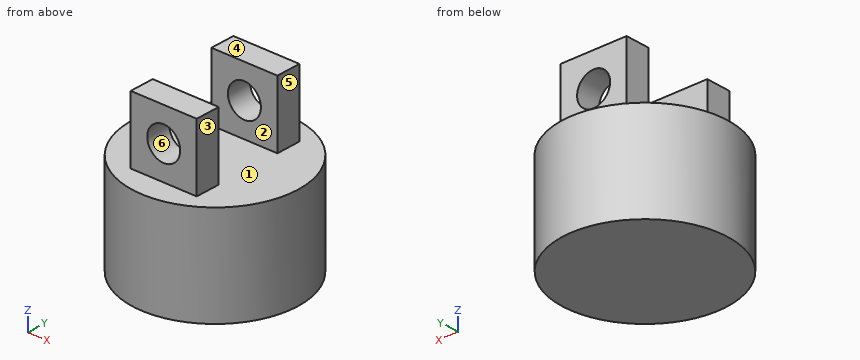
```python
from build123d import *

# Parameters (mm, degrees)
F0_R     = 31.75
F1_DEPTH = 38.1
F2_W     = 25.4
F2_H     = 9.525
F3_DEPTH = 25.4
F4_R     = 6.35
F5_DEPTH = 44.45


with BuildPart() as f1:
    # F0 (on Top) → F1 (new body)
    with BuildSketch(Plane.XY):
        Circle(F0_R)
    extrude(amount=F1_DEPTH)

    # F2 (on face) → F3 (join)
    with BuildSketch(Plane.XY.offset(38.1)):
        with Locations((0, 17.4625)):
            Rectangle(F2_W, F2_H)
        with Locations((0, -17.4625)):
            Rectangle(F2_W, F2_H)
    extrude(amount=F3_DEPTH)

    # F4 (on face) → F5 (cut, through all)
    with BuildSketch(Plane.XZ.offset(22.225)):
        with Locations((0, 50.8)):
            Circle(F4_R)
    extrude(amount=-F5_DEPTH, mode=Mode.SUBTRACT)


solid = f1.part
```
Check sheet for the modelled part. Datum: model origin and axes. Units: mm. Face numbers are marked on the shaded views. A direction names the side the tool comes from. Give positions to 0.01 mm unless a question says otherwise; leave off trailing zeros. Order: outer loops, then holes, each group sorted by start corner. A loop starts at its lowest first (then second) coordinate and runs counter-clockwise, first axis right, second up. Notation, with made-up numbers: M -27.75,-4 L 15.25,-4 A34 ccw 15.25,32 Z; hole C 9.25,15 d2. An arc over 180 degrees is marked long. Answer in a Markdown table with one row per item. Add a question column.
Q1. Access from +Z, -Z, +X, -X, +Y, -Y to the whole of each face (thin tool, end or side, straight path). Record for the marked faces 1, 2 and 3.
Q2. Gauge pin test, flat ends, axial feed: pin 1 Ø2 at (y, z) = (24, 35) entering from +X; pin 2 Ø12 at (y, z) = (7.5, 47.5) entering from +X; pin 3 Ø5 at (x, z) = (-18.5, 36.5) entering from +Y. Record the tip position at first contact, or that the pin passes through.
Q3. Release check for a two-part mould opening along Z. For the marked faces 4, 5 and 6 record: released by +Z, released by -Z, zero draft, split by the parting line, or undercut.
Q4. Sectioned sample at A-A, the plane x = 0. Record the boundary of the cut face in (y, z) (3 decimals), and give its area (3 significant figures).
Q5. Sectioned sample at D-D, the plane z = 15. Record the boundary of the cut face in (x, y), and give its area (3 significant figures).
Q6. Sectioned sample at B-B, the plane z = 50.8. Record the boundary of the cut face in (x, y) (3 decimals).
Q7. Sectioned sample at C-C, the plane y = 19. Record the boundary of the cut face in (x, z), and give its area (3 significant figures).
Q8. Thickness scan on L1, parallel to Y at x = -5.5, z = 39 (3 decimals); L2, parallel to Z at x = 0, y = -14.75; L3, parallel to Z at x = 7, y = -26.5. Record the ranges inside material, lowest first.
Verdict:
| question | item | result |
|---|---|---|
| 1 | face 1 | +Z |
| 1 | face 2 | +Z, +X, -X |
| 1 | face 3 | +Z, +X, +Y, -Y |
| 2 | pin 1 | x = 21.89 |
| 2 | pin 2 | x = 12.7 |
| 2 | pin 3 | y = 27.42 |
| 3 | face 4 | released by +Z |
| 3 | face 5 | zero draft |
| 3 | face 6 | undercut |
| 4 | outline | M -31.75,0 L 31.75,0 L 31.75,38.1 L 22.225,38.1 L 22.225,44.45 L 12.7,44.45 L 12.7,38.1 L -12.7,38.1 L -12.7,44.45 L -22.225,44.45 L -22.225,38.1 L -31.75,38.1 Z; M -22.225,57.15 L -12.7,57.15 L -12.7,63.5 L -22.225,63.5 Z; M 12.7,57.15 L 22.225,57.15 L 22.225,63.5 L 12.7,63.5 Z |
| 4 | area | 2,660 mm² |
| 5 | outline | C 0,0 d63.5 |
| 5 | area | 3,170 mm² |
| 6 | outline | M -12.7,-22.225 L -6.35,-22.225 L -6.35,-12.7 L -12.7,-12.7 Z; M -12.7,12.7 L -6.35,12.7 L -6.35,22.225 L -12.7,22.225 Z; M 6.35,-22.225 L 12.7,-22.225 L 12.7,-12.7 L 6.35,-12.7 Z; M 6.35,12.7 L 12.7,12.7 L 12.7,22.225 L 6.35,22.225 Z |
| 7 | outline | M -25.44,0 L 25.44,0 L 25.44,38.1 L 12.7,38.1 L 12.7,63.5 L -12.7,63.5 L -12.7,38.1 L -25.44,38.1 Z; hole C 0,50.8 d12.7 |
| 7 | area | 2,460 mm² |
| 8 | L1 | -22.225 to -12.7, 12.7 to 22.225 |
| 8 | L2 | 0 to 44.45, 57.15 to 63.5 |
| 8 | L3 | 0 to 38.1 |
